Read the model definition and answer for the solid it produces. Units are mm, in the model's axes. A direction names the side the tool comes from. Round coordinates to 2 decimals unless told otherwise and drop trailing zeros. Loops run counter-clockwise (first coordinate to the right, second up) from the corner with the lowest first, then second, coordinate; pieces in that order, holes last. Notation, with made-up numbers: M 84.25,36.25 L 101.25,36.25 A21 ccw 101.25,46.25 Z; hole C 57,84 d3. An arc over 180 degrees is marked long. Write each question's results on one line, items separated by ' | '.
```python
from build123d import *

# Parameters (mm, degrees)
BOSS_EXTRUDE1_DEPTH = 177.8
SKETCH2_R           = 2.38125
BOSS_EXTRUDE2_DEPTH = 2.54


with BuildPart() as part:
    # Sketch1 → Boss-Extrude1 (new body)
    with BuildSketch(Plane.XY):
        with BuildLine():
            Line((166.612434893, 69.013130193), (168.959088906, 69.985146111))
            ThreePointArc((168.959088906, 69.985146111), (179.36601208, 35.67811809), (182.88, 0))
            Line((182.88, 0), (180.34, 0))
            ThreePointArc((180.34, 0), (176.874817468, 35.182588672), (166.612434893, 69.013130193))
        make_face()
    extrude(amount=BOSS_EXTRUDE1_DEPTH)

    # Sketch2 → Boss-Extrude2 (add)
    with BuildSketch(Plane.XY.offset(177.8)):
        with BuildLine():
            Line((174.415755953, 54.993076613), (188.934873176, 59.570936689))
            ThreePointArc((188.934873176, 59.570936689), (190.885925939, 59.39393849), (192.130700085, 57.881168655))
            ThreePointArc((192.130700085, 57.881168655), (196.973310631, 38.287733012), (199.823150498, 18.306941989))
            ThreePointArc((199.823150498, 18.306941989), (199.235709562, 16.43802562), (197.493029633, 15.543038518))
            Line((197.493029633, 15.543038518), (182.316241993, 14.348599427))
            ThreePointArc((182.316241993, 14.348599427), (179.519979309, 34.895149074), (174.415755953, 54.993076613))
        make_face()
        with Locations((185.626529875, 48.001162801)):
            Circle(SKETCH2_R, mode=Mode.SUBTRACT)
        with Locations((189.904635813, 26.411162801)):
            Circle(SKETCH2_R, mode=Mode.SUBTRACT)
    boss_extrude2 = extrude(amount=-BOSS_EXTRUDE2_DEPTH)

    # Mirror1: Boss-Extrude2 across plane
    add(boss_extrude2.mirror(Plane.XY.offset(88.9)))


solid = part.part
```
1. Find the intervals of material crossed by L1, parallel to Z at x = 189, y = 45.5; L2, parallel to X at y = 62, z = 124; L3, parallel to X at y = 35.5, z = 35, in increasing order.
Completed:
L1: z = 0 to 2.54, 175.26 to 177.8 | L2: x = 169.35 to 172.05 | L3: x = 176.81 to 179.4
2. Find section A-A, the plane z = 12.5. Give the vertices of the cut face in (x, y).
Completed:
outline: M 166.61,69.01 A180.34 cw 180.34,0 L 182.88,0 A182.88 ccw 168.96,69.99 Z
3. Find section D-D, the plane y = 64. Give the vertices of the cut face in (x, z).
Completed:
outline: M 168.6,0 L 171.32,0 L 171.32,177.8 L 168.6,177.8 Z
4. Determine the mould class of faces 1 (the face through (187, 35, 177.8)), 2 (the face through (187.526, 26.516, 1.252)), 3 (the face through (187, 37, 2.54)) for opening direction Z: released by +Z, released by -Z, zero draft, split by the parting line, or undercut.
Completed:
face 1: released by +Z | face 2: zero draft | face 3: undercut
5. Find section B-B, the plane y = 35.5. Give the vertices of the cut face in (x, z), then the cut area to 3 significant figures.
Completed:
outline: M 176.81,0 L 197.49,0 L 197.49,2.54 L 179.4,2.54 L 179.4,175.26 L 197.49,175.26 L 197.49,177.8 L 176.81,177.8 Z | area: 552 mm2
6. Given P1, Ø2, axis at y = 9.5, z = 27.5, coming from the -X side; P2, Ø3, axis at x = 185.63, y = 48, coming from the -Z side; P3, Ø1, axis at y = 12.5, z = 31, coming from the +X side; P4, Ø10, axis at y = 35.5, z = 95.5, coming from the +X side, each flat-ended and moving along its own axis, determine where each tip first touches the part or whether it passes through.
Completed:
P1: stops at x = 180.03 | P2: passes through | P3: stops at x = 182.49 | P4: stops at x = 180.32
7. Which of the six approach directions +Z, -Z, +X, -X, +Y, -Y give full straight-line access (tool end or side, diameter ignored) to faces 4 (the face through (187, 37, 175.26)), 5 (the face through (196.92, 38.57, 1.25)), 6 (the face through (181.57, 57.25, 176.55))?
Completed:
face 4: +X, +Y | face 5: +Z, -Z, +X, +Y | face 6: +Z, -Z, +Y
